Autodesk Inventor part; units mm, degrees
ref_plane "YZ Plane" through (0, 0, 0) normal (1, 0, 0) x (0, 1, 0)
ref_plane "XZ Plane" through (0, 0, 0) normal (0, 1, 0) x (-1, 0, 0)
ref_plane "XY Plane" through (0, 0, 0) normal (0, 0, 1) x (1, 0, 0)
sketch "Sketch1" plane through (0, 0, 0) normal (0, 1, 0) x (-1, 0, 0)
  line L0 (0, 0) -> (12.7, 0)
  line L1 (12.7, 0) -> (12.7, -177.8)
  line L2 (12.7, -177.8) -> (0, -177.8)
  line L3 (0, -177.8) -> (0, 0)
  dimension "d0" = 12.7
  dimension "d1" = 177.8
extrude "Extrusion1" add sketch "Sketch1" along normal blind 20.574
sketch "Sketch4" plane through (0, 0, 0) normal (0, -1, 0) x (1, 0, 0)
  line L0 (0, -177.8) -> (-12.7, -177.8)
  line L1 (-12.7, -177.8) -> (0, -177.8)
  line L2 (0, -177.8) -> (0, -146.7612)
  line L3 (0, -146.7612) -> (-12.7, -146.7612)
  line L4 (-12.7, -146.7612) -> (-12.7, -177.8)
  line L5 (-12.7, -146.7612) -> (-86.3035, -127.0392)
  line L6 (-12.7, -146.7612) -> (63.5, -146.7612) construction
  line L7 (-86.3035, -127.0392) -> (-86.3035, -73.6992)
  line L8 (-86.3035, -73.6992) -> (-93.4155, -73.6992)
  line L9 (-93.4155, -73.6992) -> (-93.4155, -127.0392)
  line L10 (-12.7, -177.8) -> (0, -177.8)
  line L11 (0, -177.8) -> (0, -152.4)
  line L12 (0, -152.4) -> (-12.7, -152.4)
  line L13 (-12.7, -152.4) -> (-12.7, -177.8)
  line L14 (-12.7, -152.4) -> (-87.7132, -132.3003)
  line L15 (-87.7132, -132.3003) -> (-93.4155, -127.0392)
  point P0 (0, 0)
  dimension "d6" = 12.7
  dimension "d7" = 31.0388
  dimension "d8" = 76.2
  dimension "d9" = 165
  dimension "d10" = 53.34
  dimension "d11" = 7.112
  dimension "d12" = 12.7
  dimension "d13" = 25.4
sketch "Sketch5" plane through (-12.7, 0, -177.8) normal (-1, 0, 0) x (0, 0, 1)
  line L0 (177.8, 20.574) -> (0, 20.574)
  line L1 (0, 0) -> (177.8, 0)
  line L2 (0, 20.574) -> (31.0403, 20.574)
  line L3 (31.0403, 20.574) -> (31.0403, 0)
  line L4 (31.0403, 0) -> (0, 0)
  line L5 (0, 0) -> (0, 20.574)
  line L6 (31.0403, 10.287) -> (56.4403, 10.287)
  line L7 (56.4403, 10.287) -> (56.4403, 12.319)
  line L8 (56.4403, 12.319) -> (56.4403, 8.255)
  line L9 (56.4403, 8.255) -> (70.3595, 8.255)
  line L10 (70.3595, 8.255) -> (70.3595, 12.319)
  line L11 (70.3595, 12.319) -> (56.4403, 12.319)
  line L12 (70.3595, 12.319) -> (70.3595, 20.574)
  line L13 (70.3595, 8.255) -> (70.3595, 0)
  line L14 (70.3595, 20.574) -> (74.4235, 20.574)
  line L15 (74.4235, 20.574) -> (74.4235, 0)
  line L16 (70.3595, 0) -> (74.4235, 0)
  dimension "d14" = 25.4
  dimension "d15" = 2.032
  dimension "d16" = 4.064
  dimension "d17" = 13.9192
  dimension "d18" = 4.064
extrude "Extrusion2" add sketch "Sketch5" along normal blind 73.66 contours L15 L1 L13 L10 L12 L0 | L10 L9 L8 L7 L11
extrude "Extrusion3" add sketch "Sketch4" against normal blind 20.32 contours L14 L15 L9 L8 L7 L5 L4
sketch "Sketch6" plane through (-12.7, 0, 0) normal (-1, 0, 0) x (0, 0, 1)
  line L0 (0, 0) -> (0, 20.574)
  line L1 (0, 10.287) -> (-6.35, 10.287)
  line L2 (-6.35, 10.287) -> (-19.05, 10.287)
  circle A0 centre (-12.7, 10.287) radius 6.35
  dimension "d24" = 12.7
  dimension "d25" = 12.7
extrude "Extrusion4" cut sketch "Sketch6" against normal blind 20.32
sketch "Sketch7" plane through (0, 20.32, 0) normal (0, 1, 0) x (1, 0, 0)
  line L0 (-86.3035, 73.6992) -> (-86.3035, 103.3765)
  line L1 (-93.4155, 73.6992) -> (-86.3035, 73.6992)
  line L2 (-86.3035, 73.6992) -> (-93.4155, 73.6992)
  line L3 (-93.4155, 73.6992) -> (-93.4155, 127.0392)
  line L4 (-93.4155, 73.6992) -> (-93.4155, 127.0392)
  line L5 (-93.4155, 127.0392) -> (-87.7132, 132.3003)
  line L6 (-93.4155, 127.0392) -> (-87.7132, 132.3003)
  line L7 (-12.7, 146.7612) -> (-86.3035, 127.0392)
  line L8 (-86.3035, 73.6992) -> (-86.3035, 127.0392)
  line L9 (-86.3035, 127.0392) -> (-12.7, 146.7612)
  line L10 (-12.7, 177.8) -> (-12.7, 107.4405)
  line L11 (-12.7, 146.7612) -> (-12.7, 152.4)
  line L12 (-87.7132, 132.3003) -> (-12.7, 152.4)
  line L13 (-12.7, 152.4) -> (-87.7132, 132.3003)
  point P0 (0, 0)
  dimension "d30" = 76.2
  dimension "d31" = 5.6388
extrude "Extrusion5" add sketch "Sketch7" along normal blind 0.254
sketch "Sketch8" plane through (-93.4155, 0, -127.0392) normal (-1, 0, 0) x (0, 0, 1)
  line L0 (53.34, 0) -> (53.34, 20.574)
  line L1 (53.34, 20.574) -> (46.736, 20.574)
  line L2 (0, 20.574) -> (53.34, 20.574)
  line L3 (46.736, 20.574) -> (46.736, 0)
  line L4 (53.34, 0) -> (0, 0)
  arc A0 (46.736, 0) -> (46.736, 20.574) centre (42.026, 10.287) ccw
  point P0 (127.0392, 0)
  dimension "d34" = 6.604
extrude "Extrusion6" cut sketch "Sketch8" against normal blind 25.4 contours L4 A0 L0 | A0 L1 L0
sketch "Sketch9" plane through (-93.4155, 0, -127.0392) normal (-1, 0, 0) x (0, 0, 1)
  arc A0 (46.736, 0) -> (46.736, 20.574) centre (42.026, 10.287) ccw
  line L0 (53.34, 10.287) -> (49.276, 10.287)
  line L1 (49.276, 10.287) -> (37.2618, 10.287)
  circle A1 centre (43.2689, 10.287) radius 6.0071
  point P0 (127.0392, 0)
  dimension "d37" = 4.064
  dimension "d38" = 12.0142
extrude "Extrusion7" cut sketch "Sketch9" against normal blind 0.508
sketch "Sketch11" plane through (-92.9075, 10.287, -83.7703) normal (-1, 0, 0) x (0, 0, 1)
  circle A0 centre (0, 0) radius 4.826
  point P0 (83.7703, -10.287)
  dimension "d41" = 9.652
extrude "Extrusion8" cut sketch "Sketch11" against normal blind 22.86
sketch "Sketch12" plane through (-86.3035, 0, -103.3765) normal (1, 0, 0) x (0, 0, -1)
  circle A0 centre (-19.6062, 10.287) radius 6.0071
  circle A1 centre (-19.6062, 10.287) radius 8.89
  point P0 (-103.3765, 0)
  dimension "d44" = 17.78
extrude "Extrusion9" add sketch "Sketch12" along normal blind 16.002
sketch "Sketch13" plane through (-86.3035, 10.287, -83.7703) normal (1, 0, 0) x (0, 0, -1)
  circle A0 centre (0, 0) radius 4.826
  circle A1 centre (0, 0) radius 4.826
  circle A2 centre (0, 0) radius 6.0071
  point P0 (-83.7703, -10.287)
extrude "Extrusion10" add sketch "Sketch13" along normal blind 16.002
sketch "Sketch21" plane through (0, 0, -177.8) normal (0, 0, -1) x (-1, 0, 0)
  line L0 (0, 0) -> (12.7, 0)
  line L1 (12.7, 0) -> (12.7, 20.574)
  line L2 (12.7, 20.574) -> (0, 20.574)
  line L3 (0, 20.574) -> (0, 0)
extrude "Extrusion14" add sketch "Sketch21" along normal blind 25.4
sketch "Sketch22" plane through (-12.7, 0, -152.4) normal (-1, 0, 0) x (0, 0, 1)
  line L0 (0, 0) -> (-50.8, 0)
  line L1 (0, 20.574) -> (-50.8, 20.574)
  line L2 (-50.8, 0) -> (-25.4, 0)
  line L3 (-25.4, 0) -> (-25.4, 20.574)
  line L4 (-25.4, 20.574) -> (-50.8, 20.574)
  line L5 (-50.8, 20.574) -> (-50.8, 0)
  point P0 (152.4, 0)
extrude "Extrusion15" add sketch "Sketch22" along normal blind 2.54
properties part number "steeringBracket" material "Steel, Carbon"
The listing builds one solid part. Answer for the finished solid, in the listing's coordinates (mm). A direction names the side the tool comes from. Round coordinates to 2 decimals unless told otherwise and drop trailing zeros. Write each loop counter-clockwise with the first axis right and the second up, starting at its lowest first coordinate (ties: lowest second). Pieces come first, ordered by that corner, then holes. Notation, with made-up numbers: (82.5, -5.5) -> (107.5, -5.5) arc R3 ccw to (107.5, -1.5) -> close; hole circle Ø8 at (43.5, 76.25). An arc over 180 degrees is marked (long way). Write item = value, one per line.
1) Section A-A on z = -12.7 is taken. Write down the section's boundary in (x, y), plus the area to 4 significant figures.
Check values:
outline = (-12.7, 0) -> (0, 0) -> (0, 3.94) -> (-12.7, 3.94) -> close; (-12.7, 16.64) -> (0, 16.64) -> (0, 20.57) -> (-12.7, 20.57) -> close
area = 100.0 mm²
2) Which of the six approach directions +Z, -Z, +X, -X, +Y, -Y give full straight-line access (tool end or side, diameter ignored) to faces 4 (the flat face through (-49, 4, -107.44)), 5 (the cylindrical face through (-78.41, 7.62, -92.25)), 6 (the flat face through (-92.908, 15.2, -82.9)), 7 (the flat face through (-48.987, 10.143, -137.038))?
Check values:
face_4 = -Y
face_5 = none
face_6 = -X
face_7 = +Y, -Y
3) For a pull along X with two mould halves and no side action, classify faces 1 (the flat face through (0, 10, -100)), 2 (the flat face through (-12.7, 10, -51)), 3 (the flat face through (-93.416, 10, -100)) as released by +X, released by -X, zero draft, split by the parting line, or undercut.
Check values:
face_1 = released by +X
face_2 = undercut
face_3 = released by -X
4) Section B-B on x = -43.5 is taken. Write down the section's boundary in (y, z) (1 decimal).
Check values:
outline = (0, -144.1) -> (20.6, -144.1) -> (20.6, -138.5) -> (0, -138.5) -> close; (0, -107.4) -> (8.3, -107.4) -> (8.3, -121.4) -> (12.3, -121.4) -> (12.3, -107.4) -> (20.6, -107.4) -> (20.6, -103.4) -> (0, -103.4) -> close
5) Section C-C on z = -116 is taken. Write down the section's boundary in (x, y) (1 decimal), plus the area to 3 significant figures.
Check values:
outline = (-93.4, 0) -> (-86.3, 0) -> (-86.3, 8.3) -> (-12.7, 8.3) -> (-12.7, 0) -> (0, 0) -> (0, 20.6) -> (-12.7, 20.6) -> (-12.7, 12.3) -> (-86.3, 12.3) -> (-86.3, 20.6) -> (-93.4, 20.6) -> close
area = 707 mm²
6) Section D-D on z = -85 is taken. Write down the section's boundary in (x, y), plus the area to 3 significant figures.
Check values:
outline = (-93.42, 0) -> (-86.3, 0) -> (-86.3, 1.48) -> (-70.3, 1.48) -> (-70.3, 5.62) -> (-92.91, 5.62) -> (-92.91, 4.41) -> (-93.42, 4.41) -> close; (-93.42, 16.17) -> (-92.91, 16.17) -> (-92.91, 14.95) -> (-70.3, 14.95) -> (-70.3, 19.09) -> (-86.3, 19.09) -> (-86.3, 20.57) -> (-93.42, 20.57) -> close; (-12.7, 0) -> (0, 0) -> (0, 20.57) -> (-12.7, 20.57) -> close
area = 472 mm²
7) Given pin 1 (3.5 mm diameter, centred on y = 7.5, z = -84, fed in from -X); pin 2 (4 mm diameter, centred on x = -32.5, y = 4, fed in from -Z); pin 3 (10 mm diameter, centred on y = 10.287, z = -12.7, fed in from -X); pin 4 (6.5 mm diameter, centred on x = -55.5, y = 18, fed in from -Z), each flat-ended and moving along its own axis, determine where each tip first touches the part or whether it passes through.
Check values:
pin_1 = -12.7
pin_2 = -147.63
pin_3 = through
pin_4 = -141.8
8) Straight lines are drawn through the part: line 1 along Y through (x, z) = (-8.25, -12.7); line 2 along X through (y, z) = (9.5, -74.5); line 3 along Z through (x, y) = (-79, 6.5) (1 decimal). For each, find the intervals that lie inside material, in ascending order. Write a range as [from, to].
Check values:
line_1 = [0, 3.94], [16.64, 20.57]
line_2 = [-93.42, -86.3], [-12.7, 0]
line_3 = [-134.6, -129], [-107.4, -103.4], [-91.8, -86.8], [-80.8, -75.7]
